Verification items for the finished model (mm, model axes). Give positions to 0.01 mm unless a question says otherwise; leave off trailing zeros. Loops run counter-clockwise (first coordinate to the right, second up) from the corner with the lowest first, then second, coordinate; pieces in that order, holes last. Notation, with made-up numbers: M 59.25,12 L 98.25,12 A30 cw 98.25,37 Z; hole C 6,77.25 d4. An arc over 180 degrees is marked long. Use a Markdown table: item, result.
from build123d import *

# Parameters (mm, degrees)
SKETCH_1_W      = 55
SKETCH_1_H      = 49
SKETCH_1_R      = 1.5
EXTRUDE_1_DEPTH = 3
CHAMFER_1_SIZE  = 0.5
CHAMFER_1_SIZE2 = 0.866025404


with BuildPart() as part:
    # Эскиз1 → Бобышка-Вытянуть1 (new body)
    with BuildSketch(Plane.XY):
        with Locations((0, -3)):
            Rectangle(SKETCH_1_W, SKETCH_1_H)
        with Locations((-24.5, 15.5)):
            Circle(SKETCH_1_R, mode=Mode.SUBTRACT)
        with Locations((-24.71865387, -12.5)):
            Circle(SKETCH_1_R, mode=Mode.SUBTRACT)
        with Locations((24.5, -12.5)):
            Circle(SKETCH_1_R, mode=Mode.SUBTRACT)
        with Locations((24.430350012, 15.5)):
            Circle(SKETCH_1_R, mode=Mode.SUBTRACT)
        with Locations((0, -24.5)):
            Circle(SKETCH_1_R, mode=Mode.SUBTRACT)
    extrude(amount=EXTRUDE_1_DEPTH)

    # Фаска1
    chamfer_1_edges = [part.edges().sort_by_distance(p)[0] for p in [
        (-26, 15.5, 3),
        (-26.21865387, -12.5, 3),
        (23, -12.5, 3),
        (22.930350012, 15.5, 3),
        (-1.5, -24.5, 3),
    ]]
    chamfer_1_side = [part.faces().sort_by_distance(p)[0] for p in [
        (0.000766227, -2.990698033, 3),
    ]]
    chamfer(chamfer_1_edges, length=CHAMFER_1_SIZE, length2=CHAMFER_1_SIZE2, reference=chamfer_1_side[0])


solid = part.part
(1) Cross-section at D-D on x = -24.5. State how many separate pieces and enclosed holes the cut face has, then the cut area to 3 significant figures.
Results below:
| item | result |
|---|---|
| separate pieces | 3 |
| enclosed holes | 0 |
| area | 128 mm^2 |
(2) Material ranges on line 1 (Y direction, x = -24.5, z = 0.7); line 2 (X direction, y = -13.5, z = 2.4); line 3 (X direction, y = -24, z = 0.6), recorded low to high.
Results below:
| item | result |
|---|---|
| line 1 | -27.5 to -13.98, -11.02 to 14, 17 to 21.5 |
| line 2 | -27.5 to -26.04, -23.4 to 23.18, 25.82 to 27.5 |
| line 3 | -27.5 to -1.41, 1.41 to 27.5 |
(3) Cross-section at A-A on y = -24.5. Record the cut outline in (x, z).
Results below:
| item | result |
|---|---|
| outline | M -27.5,0 L -1.5,0 L -1.5,2.13 L -2,3 L -27.5,3 Z; M 1.5,0 L 27.5,0 L 27.5,3 L 2,3 L 1.5,2.13 Z |
(4) Cross-section at C-C on y = -12.5. Record the cut outline in (x, z), then the cut area to 3 significant figures.
Results below:
| item | result |
|---|---|
| outline | M -27.5,0 L -26.22,0 L -26.22,2.13 L -26.72,3 L -27.5,3 Z; M -23.22,0 L 23,0 L 23,2.13 L 22.5,3 L -22.72,3 L -23.22,2.13 Z; M 26,0 L 27.5,0 L 27.5,3 L 26.5,3 L 26,2.13 Z |
| area | 146 mm^2 |
(5) Draft check along Y on faces 1 (the flat face through (0, 21.5, 1)), 2 (the flat face through (0, -3, 0)), 3 (the cylindrical face through (25.86, 15.95, 1.05)). Enter one of: +Y half, -Y half, draft (parallel to the pull), parting line (faces both ways), or undercut.
Results below:
| item | result |
|---|---|
| face 1 | +Y half |
| face 2 | draft |
| face 3 | undercut |
(6) Cross-section at B-B on x = 0. Record the cut outline in (y, z).
Results below:
| item | result |
|---|---|
| outline | M -27.5,0 L -26,0 L -26,2.13 L -26.5,3 L -27.5,3 Z; M -23,0 L 21.5,0 L 21.5,3 L -22.5,3 L -23,2.13 Z |
